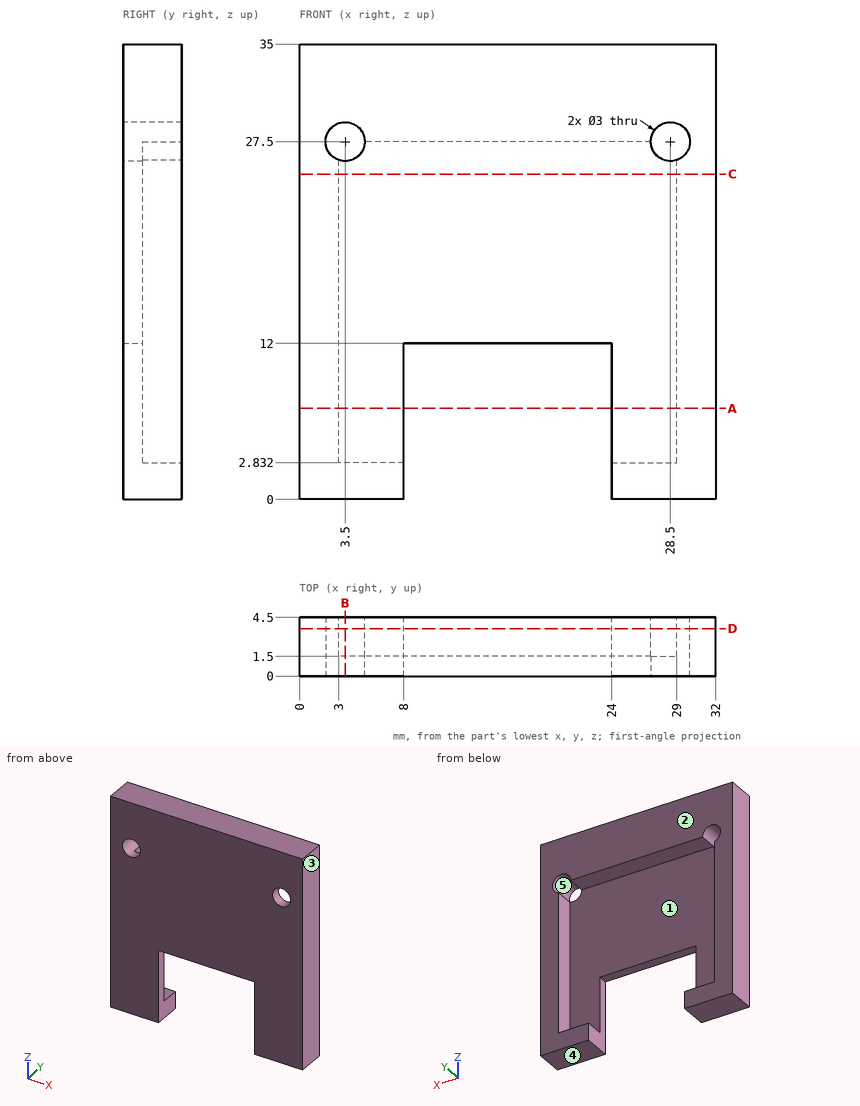
Geometry check sheet. Reference: drawing and pictorial views, mm from the part's lowest x, y, z. A direction names the side the tool comes from. Round coordinates to 2 decimals unless told otherwise and drop trailing zeros. Loops run counter-clockwise (first coordinate to the right, second up) from the corner with the lowest first, then second, coordinate; pieces in that order, holes last. Notation, with made-up numbers: (6.5, 87.25) - (61.5, 87.25) arc R14 cw to (61.5, 109.25) - close; hole circle Ø4 at (24.25, -11). An arc over 180 degrees is marked (long way). Answer as CSV lines item,"result".
(1) Cross-section at A-A, the plane z = 7. Enter the section's corners in (x, y).
Output values:
outline,"(0, 0) - (8, 0) - (8, 1.5) - (3, 1.5) - (3, 4.5) - (0, 4.5) - close; (24, 0) - (32, 0) - (32, 4.5) - (29, 4.5) - (29, 1.5) - (24, 1.5) - close"
(2) Set-up check for the marked faces 1 and 2: record each of +Z, -Z, +X, -X, +Y, -Y from which the full face is reachable in a straight line by a thin tool's end or side.
Output values:
face 1,"+Y"
face 2,"+Z, -Z, +X, -X, +Y"
(3) Material ranges on line 1 along Z through (x, y) = (28.5, 2.25); line 2 along X through (y, z) = (4.05, 5); line 3 along X through (y, z) = (1, 5), recorded low to high.
Output values:
line 1,"z = 0 to 2.83, 29 to 35"
line 2,"x = 0 to 3, 29 to 32"
line 3,"x = 0 to 8, 24 to 32"
(4) Cross-section at C-C, the plane z = 25. Enter the section's corners in (x, y).
Output values:
outline,"(0, 0) - (32, 0) - (32, 4.5) - (29, 4.5) - (29, 1.5) - (3, 1.5) - (3, 4.5) - (0, 4.5) - close"
(5) Release check for a two-part mould opening along Z. For the marked faces 3, 4 and 5 record: released by +Z, released by -Z, zero draft, split by the parting line, or undercut.
Output values:
face 3,"zero draft"
face 4,"released by -Z"
face 5,"undercut"
(6) Depth check by flat-ended pin: pin 1 Ø0.8 at (x, y) = (19.5, 0.5) entering from -Z; pin 2 Ø1.5 at (x, y) = (17, 2.5) entering from -Z; pin 3 Ø12.5 at (x, z) = (14, 11.5) entering from +Y. Enter the tip coordinate at first touch or a pass-through.
Output values:
pin 1,"stops at z = 12"
pin 2,"stops at z = 27.5"
pin 3,"stops at y = 1.5"
(7) Cross-section at D-D, the plane y = 3.65. Enter the section's corners in (x, z), and give its area (3 significant figures).
Output values:
outline,"(0, 0) - (8, 0) - (8, 2.83) - (3, 2.83) - (3, 26.09) arc R1.5 cw (long way) to (5, 27.5) - (27, 27.5) arc R1.5 cw (long way) to (29, 26.09) - (29, 2.83) - (24, 2.83) - (24, 0) - (32, 0) - (32, 35) - (0, 35) - close"
area,"424 mm²"
(8) Cross-section at B-B, the plane x = 3.5. Enter the section's corners in (y, z).
Output values:
outline,"(0, 0) - (4.5, 0) - (4.5, 2.83) - (1.5, 2.83) - (1.5, 26) - (0, 26) - close; (0, 29) - (4.5, 29) - (4.5, 35) - (0, 35) - close"
